For this review, use the dimensioned drawing (mm, ordinates from the lowest corner) and the shaded views. A direction names the side the tool comes from. Round coordinates to 2 decimals unless told otherwise and drop trailing zeros. Loops run counter-clockwise (first coordinate to the right, second up) from the corner with the lowest first, then second, coordinate; pieces in that order, holes last. Notation, with made-up numbers: (2.5, 66.25) -> (27.5, 66.25) arc R24 cw to (27.5, 103.25) -> close; hole circle Ø9 at (83.25, 69). An arc over 180 degrees is marked (long way). Answer as CSV lines item,"result". Start each with the question number.
(1) Take a section at B-B, the plane y = 5. Write out the cut boundary in (x, z), and give its area (3 significant figures).
(2) Draft analysis for pull direction X (two halves, no side actions). For the marked faces 1 and 2, state which applies: +X half, -X half, draft (parallel to the pull), parting line (faces both ways), or undercut.
(3) To check wall thickness, follow line 1 (Y direction, x = 28.44, z = 1.1); line 2 (X direction, y = 5.75, z = 1.1); line 3 (X direction, y = 5.75, z = 2). State the ranges of each line that lie inside material, in increasing order. Write a range as from..to.
(4) Take a section at A-A, the plane x = 8.44. Write out the cut boundary in (y, z).
(5) Take a section at D-D, the plane z = 0.6. Write out the cut boundary in (x, y), and give its area (3 significant figures).
(6) Take a section at C-C, the plane z = 2.3. Write out the cut boundary in (x, y).
(7) Machinability: for the marked faces 3 and 4, which of the approach directions +Z, -Z, +X, -X, +Y, -Y give a long, thin tool a straight path to every point of the face, cutting with its end or side? Answer none if there is none.
(8) For P1, Ø1, axis at x = 8, z = 2.5, coming from the +Y side, flat-tipped, find the tip position at first contact; note if it passes through.
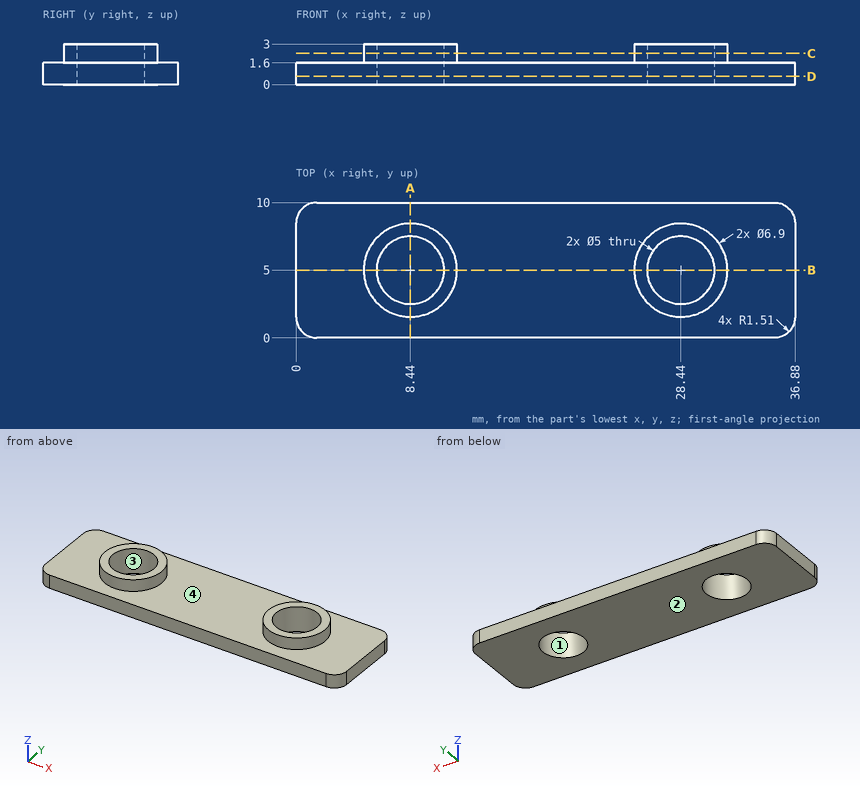
The answers:
1,outline,"(0, 0) -> (5.94, 0) -> (5.94, 3) -> (4.99, 3) -> (4.99, 1.6) -> (0, 1.6) -> close; (10.94, 0) -> (25.94, 0) -> (25.94, 3) -> (24.99, 3) -> (24.99, 1.6) -> (11.89, 1.6) -> (11.89, 3) -> (10.94, 3) -> close; (30.94, 0) -> (36.88, 0) -> (36.88, 1.6) -> (31.89, 1.6) -> (31.89, 3) -> (30.94, 3) -> close"
1,area,"48.3 mm²"
2,face 1,"undercut"
2,face 2,"draft"
3,line 1,"0..2.5, 7.5..10"
3,line 2,"0..6.06, 10.82..26.06, 30.82..36.88"
3,line 3,"5.07..6.06, 10.82..11.81, 25.07..26.06, 30.82..31.81"
4,outline,"(0, 0) -> (2.5, 0) -> (2.5, 3) -> (1.55, 3) -> (1.55, 1.6) -> (0, 1.6) -> close; (7.5, 0) -> (10, 0) -> (10, 1.6) -> (8.45, 1.6) -> (8.45, 3) -> (7.5, 3) -> close"
5,outline,"(0, 1.51) arc R1.51 ccw to (1.51, 0) -> (35.37, 0) arc R1.51 ccw to (36.88, 1.51) -> (36.88, 8.49) arc R1.51 ccw to (35.37, 10) -> (1.51, 10) arc R1.51 ccw to (0, 8.49) -> close; hole circle Ø5 at (8.44, 5); hole circle Ø5 at (28.44, 5)"
5,area,"328 mm²"
6,outline,"circle Ø6.9 at (8.44, 5); circle Ø6.9 at (28.44, 5); hole circle Ø5 at (8.44, 5); hole circle Ø5 at (28.44, 5)"
7,face 3,"+Z, -Z"
7,face 4,"+Z"
8,P1,"y = 8.45"
